Input: part model. Units: mm. Frame: model coordinates. A direction names the side the tool comes from. Round coordinates to 2 decimals unless told otherwise and drop trailing zeros. Loops run counter-clockwise (first coordinate to the right, second up) from the corner with the lowest first, then second, coordinate; pieces in that order, holes last. Notation, with made-up numbers: (50.25, -3.75) -> (100.25, -3.75) arc R18 ccw to (100.25, 20.25) -> close; hole circle Ø3 at (-4.5, 22). An arc over 180 degrees is marked (long way). Answer as a JSON object with one key per item and string values. Group by question number.
Item 1: Section query C-C on x = -37.5. Return loops of the section in (y, z), and give its area (3 significant figures).
Item 2: Pin query (flat end, axial travel): pin 1 (3 mm diameter, centred on y = -32, z = 20, fed in from -X); pin 2 (10 mm diameter, centred on y = -11.5, z = 31, fed in from -X); pin 3 (12 mm diameter, centred on x = 5.5, y = -33.5, fed in from +Z). Return the tip coordinate at first contact, or that it passes through.
Item 3: Draft query along Z for faces 4 (the flat face through (-47.691, -20.912, 7.205)), 5 (the flat face through (-48.7, -18, 16)), 6 (the flat face through (43.09, -20.91, 19.76)). Return one class per face: released by +Z, released by -Z, zero draft, split by the parting line, or undercut.
Item 4: Section query B-B on y = -15. Return loops of the section in (x, z), and give its area (3 significant figures).
Item 5: Section query A-A on z = 20.5. Return loops of the section in (x, y), and give its area (3 significant figures).
Item 6: Set-up query: faces 1 (the flat face through (1, -42.418, 14)), 2 (the flat face through (-16.361, -20.912, 23.425)), 3 (the flat face through (-46, -0.762, 26)). Return all of +Z, -Z, +X, -X, +Y, -Y with unobstructed straight access to the full face (end or side cutting, diameter ignored); none if empty.
Item 7: Section query D-D on z = 8. Return loops of the section in (x, y), and give its area (3 significant figures).
Item 8: Material intervals for line 1 (Z direction, x = 7, y = -15.5); line 2 (Z direction, x = -33.5, y = -2.5); line 3 (X direction, y = -10, z = 15), sorted ascending. Write a range as [from, to].
from build123d import *

# Parameters (mm, degrees)
F1_DEPTH = 42.418
F3_DEPTH = 42.672
F4_DEPTH = 1.016


with BuildPart() as f1:
    # F0 (on Front) → F1 (new body)
    with BuildSketch(Plane.XZ):
        Polygon((0, 18.5649488121), (-33.1869013608, 28.4224450588), (-50.9303919971, 14.2112225294), (-44.3587265909, 0), (51.8207407387, 0), (58.1592172384, 11.3361189142), (27.600986883, 28.4224450588), align=None)
    extrude(amount=F1_DEPTH)

    # F2 (on face) → F3 (join)
    with BuildSketch(Plane.XZ.offset(42.418)):
        with BuildLine():
            ThreePointArc((-33.1869013608, 28.4224450588), (-39.2604604224, 31.3968249678), (-44.0265255123, 36.194707738))
            ThreePointArc((-44.0265255123, 36.194707738), (-53.7891889284, 27.8738262503), (-48.4137057273, 16.2269019326))
            Line((-48.4137057273, 16.2269019326), (-33.1869013608, 28.4224450588))
        make_face()
    extrude(amount=-F3_DEPTH)

    # F4 (cut): a face of the model
    f4_faces = [f1.faces().sort_by_distance(p)[0] for p in [
        (-45.7791341784, 0.254, 26.7092590305),
    ]]
    extrude(f4_faces, amount=-F4_DEPTH, mode=Mode.SUBTRACT)


solid = f1.part
Solved:
{
 "1": {"outline": "(-42.42, 0) -> (0, 0) -> (0, 24.97) -> (-0.76, 24.97) -> (-0.76, 30.27) -> (-42.42, 30.27) -> close", "area": "1,280 mm²"},
 "2": {"pin 1": "x = -53.21", "pin 2": "x = -54.03", "pin 3": "z = 22.67"},
 "3": {"face 4": "released by -Z", "face 5": "undercut", "face 6": "released by +Z"},
 "4": {"outline": "(-50.93, 14.21) -> (-44.36, 0) -> (51.82, 0) -> (58.16, 11.34) -> (27.6, 28.42) -> (0, 18.56) -> (-33.19, 28.42) arc R20.38 cw to (-44.03, 36.19) arc R10.62 ccw to (-48.41, 16.23) -> close", "area": "2,560 mm²"},
 "5": {"outline": "(-52.73, -42.42) -> (-6.51, -42.42) -> (-6.51, 0) -> (-43.08, 0) -> (-43.08, -0.76) -> (-52.73, -0.76) -> close; (5.42, -42.42) -> (41.77, -42.42) -> (41.77, 0) -> (5.42, 0) -> close", "area": "3,500 mm²"},
 "6": {"face 1": "+Z, -Z, +X, -X, -Y", "face 2": "+Z, +Y, -Y", "face 3": "+Z, -X, +Y"},
 "7": {"outline": "(-48.06, -42.42) -> (56.29, -42.42) -> (56.29, 0) -> (-48.06, 0) -> close", "area": "4,430 mm²"},
 "8": {"line 1": "[0, 21.06]", "line 2": "[0, 28.52]", "line 3": "[-49.95, 51.61]"}
}
